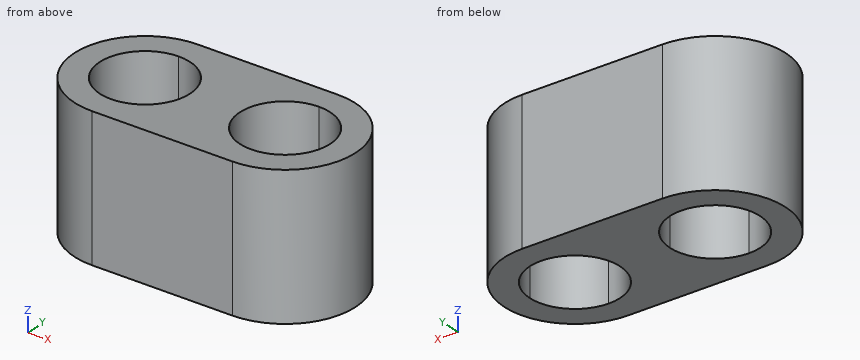
from build123d import *

# Parameters (mm, degrees)
F1_DEPTH = 7.9375


with BuildPart() as f1:
    # F0 (on Top) → F1 (new body)
    with BuildSketch(Plane.XY):
        with BuildLine():
            Line((7.9375, 3.96875), (0, 3.96875))
            Line((0, 3.96875), (0, 2.54))
            ThreePointArc((0, 2.54), (1.796051, 1.796051), (2.54, 0))
            ThreePointArc((2.54, 0), (1.796051, -1.796051), (0, -2.54))
            Line((0, -2.54), (0, -3.96875))
            Line((0, -3.96875), (7.9375, -3.96875))
            Line((7.9375, -3.96875), (7.9375, -2.54))
            ThreePointArc((7.9375, -2.54), (5.3975, 0), (7.9375, 2.54))
            Line((7.9375, 2.54), (7.9375, 3.96875))
        make_face()
        with BuildLine():
            Line((0, 2.54), (0, 3.96875))
            ThreePointArc((0, 3.96875), (-3.96875, 0), (0, -3.96875))
            Line((0, -3.96875), (0, -2.54))
            ThreePointArc((0, -2.54), (-2.54, 0), (0, 2.54))
        make_face()
        with BuildLine():
            ThreePointArc((7.9375, -3.96875), (11.90625, 0), (7.9375, 3.96875))
            Line((7.9375, 3.96875), (7.9375, 2.54))
            ThreePointArc((7.9375, 2.54), (9.733551, 1.796051), (10.4775, 0))
            ThreePointArc((10.4775, 0), (9.733551, -1.796051), (7.9375, -2.54))
            Line((7.9375, -2.54), (7.9375, -3.96875))
        make_face()
    extrude(amount=F1_DEPTH)


solid = f1.part
CAD build for the part. Positions are in the model's coordinates, mm. Round coordinates to 2 decimals unless told otherwise and drop trailing zeros. Order: outer loops, then holes, each group sorted by start corner. A loop starts at its lowest first (then second) coordinate and runs counter-clockwise, first axis right, second up. Notation, with made-up numbers: (-2.75, -32) -> (40.25, -32) arc R10 cw to (40.25, -14) -> close; hole circle Ø8 at (14.25, 48). An arc over 180 degrees is marked (long way). Write each question's results on one line, items separated by ' | '.
1. Cut at D-D (x = 9.5). Give the cut face in (y, z), plus the area to 3 significant figures.
Findings below:
outline: (-3.65, 0) -> (-2, 0) -> (-2, 7.94) -> (-3.65, 7.94) -> close; (2, 0) -> (3.65, 0) -> (3.65, 7.94) -> (2, 7.94) -> close | area: 26.1 mm²
2. Cut at A-A (z = 6). Give the cut face in (x, y).
Findings below:
outline: (0, -3.97) -> (7.94, -3.97) arc R3.97 ccw to (7.94, 3.97) -> (0, 3.97) arc R3.97 ccw to start; hole (0, 2.54) arc R2.54 ccw (long way) to (2.54, 0) arc R2.54 ccw to start; hole (7.94, 2.54) arc R2.54 ccw (long way) to (10.48, 0) arc R2.54 ccw to start
3. Cut at C-C (y = -1). Give the cut face in (x, z), plus the area to 3 significant figures.
Findings below:
outline: (-3.84, 0) -> (-2.33, 0) -> (-2.33, 7.94) -> (-3.84, 7.94) -> close; (2.33, 0) -> (5.6, 0) -> (5.6, 7.94) -> (2.33, 7.94) -> close; (10.27, 0) -> (11.78, 0) -> (11.78, 7.94) -> (10.27, 7.94) -> close | area: 49.8 mm²
4. Wall check: line 1 along X through (y, z) = (-0.5, 3.5); line 2 along X through (y, z) = (1, 4); line 3 along Y through (x, z) = (9, 0.5). Give the ranges that are in metal, low to high. Write a range as [from, to].
Findings below:
line 1: x = [-3.94, -2.49], [2.49, 5.45], [10.43, 11.87] | line 2: x = [-3.84, -2.33], [2.33, 5.6], [10.27, 11.78] | line 3: y = [-3.82, -2.31], [2.31, 3.82]
5. Flat gauge pin, fed straight in: P1, Ø2, axis at y = -3, z = 4.5, coming from the +X side. Where does the tip first touch, or does it go through?
Findings below:
P1: stops at x = 11.37
6. Cut at B-B (x = 0.5). Give the cut face in (y, z), plus the area to 3 significant figures.
Findings below:
outline: (-3.97, 0) -> (-2.49, 0) -> (-2.49, 7.94) -> (-3.97, 7.94) -> close; (2.49, 0) -> (3.97, 0) -> (3.97, 7.94) -> (2.49, 7.94) -> close | area: 23.5 mm²
